Could you check a few things on this model? Use its own coordinates, in mm. Give positions to 0.01 mm unless a question says otherwise; leave off trailing zeros. Loops run counter-clockwise (first coordinate to the right, second up) from the corner with the lowest first, then second, coordinate; pieces in that order, holes last. Notation, with made-up numbers: (45.25, 79) - (72.25, 79) arc R25 cw to (72.25, 105) - close; hole circle Ø7 at (82.5, 78). An arc over 180 degrees is marked (long way). Write each question's results on one line, items separated by ' | '. Start each with the question number.
(1) I need wall thicknesses on line 1 (X direction, y = -24, z = -2.5); line 2 (X direction, y = -10, z = -2.25); line 3 (Y direction, x = 14, z = -1.5). Which ranges of each line are inside material? Lowest first, please.
(2) Suppose I cut it at A-A (y = 12). Please give me the cut outline in (x, z).
(3) For pin 1 (1.5 mm diameter, centred on y = 3, z = -1, fed in from -X); pin 2 (0.9 mm diameter, centred on y = -10.5, z = -2, fed in from +X); pin 3 (2.5 mm diameter, centred on x = -50.34, y = 19.91, fed in from +Z), each with a flat end and sliding along its axis, tell me the tip position at first contact or that it passes through.
(4) Suppose I cut it at B-B (x = -18.5). Please give me the cut outline in (y, z).
(5) Suppose I cut it at C-C (z = -1.05). Please give me the cut outline in (x, y), and give its area (3 significant figures).
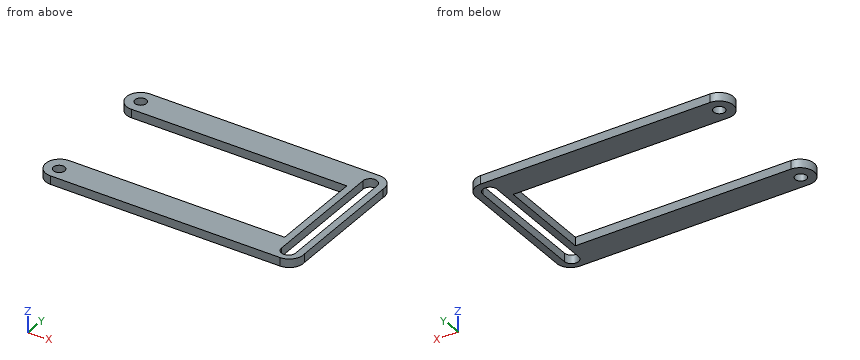
from build123d import *

# Parameters (mm, degrees)
SKETCH_1_R          = 2
EXTRUDE_1_DEPTH     = 3
SKETCH_6_R          = 2
CUT_EXTRUDE_1_DEPTH = 6
CUT_EXTRUDE_2_DEPTH = 6


with BuildPart() as part:
    # 草图1 → 凸台-拉伸1 (new body)
    with BuildSketch(Plane.XY):
        with BuildLine():
            Line((30.750249224, 24.910133645), (-50.336395226, 24.910133645))
            ThreePointArc((-50.336395226, 24.910133645), (-55.336395226, 19.910133645), (-50.336395226, 14.910133645))
            Line((-50.336395226, 14.910133645), (25.802071198, 14.910133645))
            Line((25.802071198, 14.910133645), (25.802071198, -18.575080464))
            Line((25.802071198, -18.575080464), (-50.336395226, -18.575080464))
            ThreePointArc((-50.336395226, -18.575080464), (-55.336395226, -23.575080464), (-50.336395226, -28.575080464))
            Line((-50.336395226, -28.575080464), (30.750249224, -28.575080464))
            ThreePointArc((30.750249224, -28.575080464), (34.531124493, -26.846927374), (35.69842725, -22.857073344))
            Line((35.69842725, -22.857073344), (35.69842725, 19.192126526))
            ThreePointArc((35.69842725, 19.192126526), (34.531124493, 23.181980555), (30.750249224, 24.910133645))
        make_face()
        with Locations((-50.336395226, 19.910133645)):
            Circle(SKETCH_1_R, mode=Mode.SUBTRACT)
    extrude(amount=-EXTRUDE_1_DEPTH)

    # 草图6 → 切除-拉伸1 (cut)
    with BuildSketch(Plane.XY):
        with Locations((-50.336395226, -23.991463112)):
            Circle(SKETCH_6_R)
    extrude(amount=-CUT_EXTRUDE_1_DEPTH, mode=Mode.SUBTRACT)

    # 草图13 → 切除-拉伸2 (cut)
    with BuildSketch(Plane.XY):
        with BuildLine():
            Line((33.24842725, 19.910133645), (33.24842725, -23.991463112))
            ThreePointArc((33.24842725, -23.991463112), (30.750249224, -26.489641138), (28.252071198, -23.991463112))
            Line((28.252071198, -23.991463112), (28.252071198, 19.910133645))
            ThreePointArc((28.252071198, 19.910133645), (30.750249224, 22.408311671), (33.24842725, 19.910133645))
        make_face()
    extrude(amount=-CUT_EXTRUDE_2_DEPTH, mode=Mode.SUBTRACT)


solid = part.part
Output values:
1) line 1: -55.32 to -52.34, -48.34 to 28.25, 33.25 to 35.73 | line 2: 25.8 to 28.25, 33.25 to 35.7 | line 3: -28.58 to -18.58, 14.91 to 24.91
2) outline: (25.8, -3) - (28.25, -3) - (28.25, 0) - (25.8, 0) - close; (33.25, -3) - (35.7, -3) - (35.7, 0) - (33.25, 0) - close
3) pin 1: x = 25.8 | pin 2: x = 35.7 | pin 3: through
4) outline: (-28.58, -3) - (-18.58, -3) - (-18.58, 0) - (-28.58, 0) - close; (14.91, -3) - (24.91, -3) - (24.91, 0) - (14.91, 0) - close
5) outline: (-50.34, -28.58) - (30.75, -28.58) arc R5 ccw to (35.7, -22.86) - (35.7, 19.19) arc R5 ccw to (30.75, 24.91) - (-50.34, 24.91) arc R5 ccw to (-50.34, 14.91) - (25.8, 14.91) - (25.8, -18.58) - (-50.34, -18.58) arc R5 ccw to start; hole circle Ø4 at (-50.34, -23.99); hole circle Ø4 at (-50.34, 19.91); hole (28.25, -23.99) arc R2.5 ccw to (33.25, -23.99) - (33.25, 19.91) arc R2.5 ccw to (28.25, 19.91) - close | area: 1,860 mm2
